Build history of the part. All positions in model axes, mm. Give positions to 0.01 mm unless a question says otherwise; leave off trailing zeros. Order: outer loops, then holes, each group sorted by start corner. A loop starts at its lowest first (then second) coordinate and runs counter-clockwise, first axis right, second up. Notation, with made-up numbers: (37.25, 76) -> (72.25, 76) arc R25 cw to (72.25, 103) -> close; hole circle Ø7 at (-13, 16). An arc over 180 degrees is marked (long way). One line per item, written item: value. Start each with the question number.
(1) Two-plate mould, pull along Y, no slides. Class faces 1 (the cylindrical face through (-2.579, 1.978, 2.465)), 2 (the flat face through (1, -2, 5)), 3 (the cylindrical face through (0, 2, 2)): +Y half, -Y half, draft (parallel to the pull), parting line (faces both ways), or undercut.
(2) Probe line 1 (X direction, y = 0, z = 2.65); line 2 (X direction, y = -0.75, z = 1.6). List the from-to ranges inside material, lowest first.
(3) Saw through at D-D on y = 2.25. Give the cut face in (x, z), plus the area to 3 significant figures.
(4) Saw through at A-A on x = 0. Give the cut face in (y, z).
(5) Saw through at C-C on z = 4.5. Give the cut face in (x, y).
Autodesk Fusion 360 part; units mm, degrees
sketch "Sketch1" plane through (0, 0, 0) normal (0, 0, 1) x (1, 0, 0)
  circle A0 centre (0, 0) radius 2
  circle A1 centre (0, 0) radius 2.75
  dimension "d5" = 4
  dimension "d8" = 5.5
extrude "Extrude2" add sketch "Sketch1" along normal blind 6.6
move_face "OffsetFaces1" offset 0.5 1 faces at (2.7466, -0.1371, 4.4)
extrude "Extrude3" cut 1 faces at (2.8212, 0.1615, 6.6) along direction (0, 0, -1) blind 1.6
Results below:
1. face 1: parting line
1. face 2: draft
1. face 3: undercut
2. line 1: x = -3.25 to -2, 2 to 3.25
2. line 2: x = -3.16 to -1.85, 1.85 to 3.16
3. outline: (-2.35, 0) -> (2.35, 0) -> (2.35, 5) -> (-2.35, 5) -> close
3. area: 23.5 mm²
4. outline: (-3.25, 0) -> (-2, 0) -> (-2, 5) -> (-3.25, 5) -> close; (2, 0) -> (3.25, 0) -> (3.25, 5) -> (2, 5) -> close
5. outline: circle Ø6.5 at (0, 0); hole circle Ø4 at (0, 0)
